from build123d import *

# Parameters (mm, degrees)
BOSS_EXTRUDE2_DEPTH = 2.7
SKETCH2_RX          = 1.5
SKETCH2_RY          = 1.448888739
SKETCH2_RX_2        = 4
SKETCH2_RY_2        = 3.863703305
SKETCH2_W           = 2.7
SKETCH2_H           = 19.318516525
CUT_EXTRUDE1_DEPTH  = 3


with BuildPart() as part:
    # Sketch1 → Boss-Extrude2 (new body)
    with BuildSketch(Plane(origin=(0, 0, 0), x_dir=(1, 0, 0), z_dir=(0, 1, 0))):
        Polygon((-80, -98.5), (80, -98.5), (80, -88.5), (82.7, -88.5), (82.7, -78.5), (80, -78.5), (80, -68.5), (82.7, -68.5), (82.7, -58.5), (80, -58.5), (80, -48.5), (82.7, -48.5), (82.7, -38.5), (80, -38.5), (80, -28.5), (82.7, -28.5), (82.7, -18.5), (80, -18.5), (80, -8.5), (82.7, -8.5), (82.7, 1.5), (80, 1.5), (80, 11.5), (82.7, 11.5), (82.7, 21.5), (80, 21.5), (80, 31.5), (82.7, 31.5), (82.7, 41.5), (80, 41.5), (80, 51.5), (82.7, 51.5), (82.7, 61.5), (80, 61.5), (80, 71.5), (82.7, 71.5), (82.7, 81.5), (80, 81.5), (80, 98.5), (-80, 98.5), (-80, 81.5), (-82.7, 81.5), (-82.7, 71.5), (-80, 71.5), (-80, 61.5), (-82.7, 61.5), (-82.7, 51.5), (-80, 51.5), (-80, 41.5), (-82.7, 41.5), (-82.7, 31.5), (-80, 31.5), (-80, 21.5), (-82.7, 21.5), (-82.7, 11.5), (-80, 11.5), (-80, 1.5), (-82.7, 1.5), (-82.7, -8.5), (-80, -8.5), (-80, -18.5), (-82.7, -18.5), (-82.7, -28.5), (-80, -28.5), (-80, -38.5), (-82.7, -38.5), (-82.7, -48.5), (-80, -48.5), (-80, -58.5), (-82.7, -58.5), (-82.7, -68.5), (-80, -68.5), (-80, -78.5), (-82.7, -78.5), (-82.7, -88.5), (-80, -88.5), align=None)
    extrude(amount=BOSS_EXTRUDE2_DEPTH)

    # Sketch2 → Cut-Extrude1 (cut)
    with BuildSketch(Plane(origin=(0, 2.7, 0), x_dir=(1, 0, 0), z_dir=(0, 1, 0))):
        with Locations((8.1925, 15.347700679)):
            Ellipse(SKETCH2_RX, SKETCH2_RY)
        with Locations((0, 15.347700679)):
            Ellipse(SKETCH2_RX_2, SKETCH2_RY_2)
        with Locations(Location((-8.1925, 15.347700679), (0, 0, 180))):
            Ellipse(SKETCH2_RX, SKETCH2_RY)
        with Locations((26.35, 15.347700679)):
            Rectangle(SKETCH2_W, SKETCH2_H)
        with Locations((-26.35, 15.347700679)):
            Rectangle(SKETCH2_W, SKETCH2_H)
    extrude(amount=-CUT_EXTRUDE1_DEPTH, mode=Mode.SUBTRACT)


solid = part.part
Part model, mm, in its own coordinate system. Give positions to 0.01 mm unless a question says otherwise; leave off trailing zeros. Loops run counter-clockwise (first coordinate to the right, second up) from the corner with the lowest first, then second, coordinate; pieces in that order, holes last. Notation, with made-up numbers: M -31.5,22 L 5.5,22 A24 ccw 5.5,47 Z; hole C 20.5,69.25 d4. An arc over 180 degrees is marked long. Put each result on its own line as item: value. Start each with the question number.
1) Probe probe 1 along X at (y, z) = (2.4, -7); probe 2 along X at (y, z) = (1.55, -66); probe 3 along X at (y, z) = (1.5, -12). List the from-to ranges inside material, lowest first.
2) Saw through at B-B (y = 1.55). State how many separate pieces and enclosed holes the cut face has, then the cut area to 3 significant figures.
3) Flat gauge pins, fed straight in: pin 1 (1.4 mm diameter, centred on y = 1.5, z = -7, fed in from -X); pin 2 (1.4 mm diameter, centred on x = 82, y = 1, fed in from +Z); pin 3 (0.8 mm diameter, centred on x = -82, y = 1, fed in from -Z). Where does each tip first touch, or does it go through?
4) Saw through at A-A (z = 32). List the corners of the cut face in (x, y).
Numbers:
1. probe 1: -80 to -27.7, -25 to 25, 27.7 to 80
1. probe 2: -80 to 80
1. probe 3: -82.7 to -27.7, -25 to -2, 2 to 25, 27.7 to 82.7
2. separate pieces: 1
2. enclosed holes: 5
2. area: 31,800 mm^2
3. pin 1: x = -80
3. pin 2: z = 88.5
3. pin 3: z = -81.5
4. outline: M -80,0 L 80,0 L 80,2.7 L -80,2.7 Z
